```python
from build123d import *

# Parameters (mm, degrees)
F0_W           = 42.460177
F0_H           = 28.017944
F1_DEPTH       = 25.4
F3_D           = 13.74
F3_CBORE_D     = 19.2
F3_CBORE_DEPTH = 14
F4_W           = 42.460177
F4_H           = 2.585244
F5_DEPTH       = 4


with BuildPart() as f1:
    # F0 (on Top) → F1 (new body)
    with BuildSketch(Plane.XY):
        with Locations((-26.357082, 24.479595)):
            Rectangle(F0_W, F0_H)
    extrude(amount=F1_DEPTH)

    # F3 (through all)
    with Locations(Plane.XY.offset(25.4)):
        with Locations((-27.221344, 23.667647)):
            CounterBoreHole(F3_D / 2, F3_CBORE_D / 2, F3_CBORE_DEPTH)

    # F4 (on face) → F5 (join)
    with BuildSketch(Plane(origin=(0, 38.488567, 0), x_dir=(-1, 0, 0), z_dir=(0, 1, 0))):
        with Locations((26.357082, 24.107378)):
            Rectangle(F4_W, F4_H)
    extrude(amount=F5_DEPTH)


solid = f1.part
```
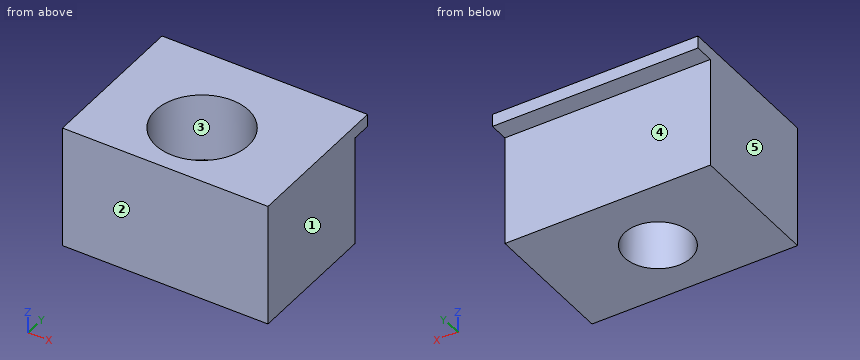
Here's how the part is built. I have some questions about the finished solid (model axes, mm). Face numbers are marked on the shaded views. A direction names the side the tool comes from. Round coordinates to 2 decimals unless told otherwise and drop trailing zeros. Loops run counter-clockwise (first coordinate to the right, second up) from the corner with the lowest first, then second, coordinate; pieces in that order, holes last.
1. Thinking about a two-plate mould opening in X: for the marked faces 1, 2 and 3, which applies, released by +X, released by -X, zero draft, split by the parting line, or undercut?
Answers:
face 1: released by +X
face 2: zero draft
face 3: undercut
2. Suppose I cut it at D-D, the plane x = -35. Please give me the cut outline in (y, z).
Answers:
outline: (10.47, 0) - (38.49, 0) - (38.49, 22.81) - (42.49, 22.81) - (42.49, 25.4) - (29.29, 25.4) - (29.29, 11.4) - (18.04, 11.4) - (18.04, 25.4) - (10.47, 25.4) - close
3. Suppose I cut it at B-B, the plane y = 28.5. Please give me the cut outline in (x, z).
Answers:
outline: (-47.59, 0) - (-32.1, 0) - (-32.1, 11.4) - (-35.52, 11.4) - (-35.52, 25.4) - (-47.59, 25.4) - close; (-22.34, 0) - (-5.13, 0) - (-5.13, 25.4) - (-18.93, 25.4) - (-18.93, 11.4) - (-22.34, 11.4) - close
4. For the marked faces 4 and 5, which set-ups out of +Z, -Z, +X, -X, +Y, -Y let a thin tool reach every point of the face, with its end or its side?
Answers:
face 4: -Z, +X, -X, +Y
face 5: +Z, -Z, -X, +Y, -Y
5. Suppose I cut it at A-A, the plane x = -23.5. Please give me the cut outline in (y, z).
Answers:
outline: (10.47, 0) - (17.89, 0) - (17.89, 11.4) - (14.82, 11.4) - (14.82, 25.4) - (10.47, 25.4) - close; (29.44, 0) - (38.49, 0) - (38.49, 22.81) - (42.49, 22.81) - (42.49, 25.4) - (32.52, 25.4) - (32.52, 11.4) - (29.44, 11.4) - close
6. Suppose I cut it at C-C, the plane z = 15. Please give me the cut outline in (x, y), and give its area (3 significant figures).
Answers:
outline: (-47.59, 10.47) - (-5.13, 10.47) - (-5.13, 38.49) - (-47.59, 38.49) - close; hole circle Ø19.2 at (-27.22, 23.67)
area: 900 mm2
7. If I drill on probe 1 along Y at (x, z) = (-27, 7); probe 2 along Y at (x, z) = (-16, 2.5); probe 3 along X at (y, z) = (27.5, 13.5), over which ranges is the centre line in solid material (lowest first)?
Answers:
probe 1: y = 10.47 to 16.8, 30.53 to 38.49
probe 2: y = 10.47 to 38.49
probe 3: x = -47.59 to -36.02, -18.42 to -5.13
8. Will these pins go through, and if not, where does the flat tip stop? pin 1 (1.5 mm diameter, centred on x = -25.5, z = 18, fed in from +Y); pin 2 (6 mm diameter, centred on x = -22.5, y = 20.5, fed in from -Z); pin 3 (12.5 mm diameter, centred on x = -27.22, y = 23.67, fed in from +Z).
Answers:
pin 1: stops at y = 38.49
pin 2: stops at z = 0
pin 3: passes through
